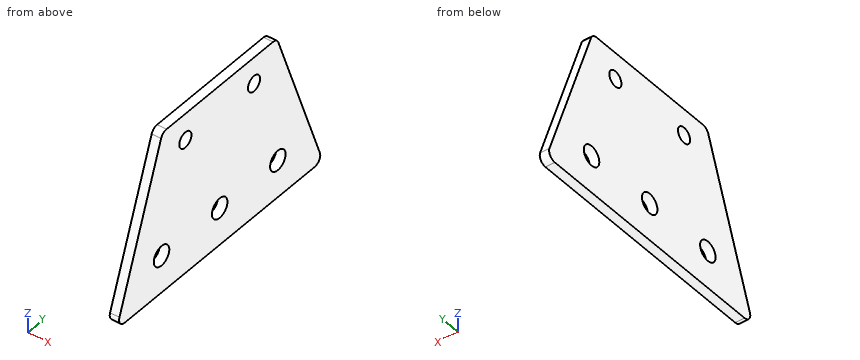
```python
from build123d import *

# Parameters (mm, degrees)
F_1_8_INCH_SHEET_DEPTH     = 1.5875
M5_CLEARANCE_HOLE1_D       = 5.3
F_1_4_IN_CLEARANCE_HOLE1_D = 6.7564
FILLET1_R                  = 2.5


with BuildPart() as part:
    # Sketch1 → 1/8 Inch Sheet (new, symmetric)
    with BuildSketch(Plane(origin=(0, 0, 0), x_dir=(0, 0, -1), z_dir=(1, 0, 0))):
        Polygon((-27.5, 25), (-27.5, -25), (27.5, -45), (27.5, 45), align=None)
    extrude(amount=F_1_8_INCH_SHEET_DEPTH, both=True)

    # M5 Clearance Hole1 (through all)
    with Locations(Plane(origin=(1.5875, 0, 0), x_dir=(0, 0, -1), z_dir=(1, 0, 0))):
        with Locations((-18.5, 15), (-18.5, -15)):
            Hole(M5_CLEARANCE_HOLE1_D / 2)

    # 1/4 in Clearance Hole1 (through all)
    with Locations(Plane(origin=(1.5875, 0, 0), x_dir=(0, 0, -1), z_dir=(1, 0, 0))):
        with Locations((14.8, 25.4), (14.8, 0), (14.8, -25.4)):
            Hole(F_1_4_IN_CLEARANCE_HOLE1_D / 2)

    # Fillet1
    fillet1_edges = [part.edges().sort_by_distance(p)[0] for p in [
        (0, 45, -27.5),
        (0, -45, -27.5),
        (0, -25, 27.5),
        (0, 25, 27.5),
    ]]
    fillet(fillet1_edges, radius=FILLET1_R)


solid = part.part
```
The listing builds one solid part. Answer for the finished solid, in the listing's coordinates (mm). Give positions to 0.01 mm unless a question says otherwise; leave off trailing zeros. Order: outer loops, then holes, each group sorted by start corner. A loop starts at its lowest first (then second) coordinate and runs counter-clockwise, first axis right, second up. Notation, with made-up numbers: (62, -2) -> (89, -2) arc R10 cw to (89, 6) -> close; hole circle Ø5 at (-25, 23.25). An arc over 180 degrees is marked (long way). Write each question's results on one line, items separated by ' | '.
Q1. The part is cut by section A-A, the plane y = -15. Give the vertices of the cut face in (x, z).
Checked values:
outline: (-1.59, -27.5) -> (1.59, -27.5) -> (1.59, 15.85) -> (-1.59, 15.85) -> close; (-1.59, 21.15) -> (1.59, 21.15) -> (1.59, 27.5) -> (-1.59, 27.5) -> close
Q2. Straight lines are drawn through the part: probe 1 along Y at (x, z) = (0, 20.5); probe 2 along Y at (x, z) = (0.45, -14.8); probe 3 along Y at (x, z) = (0.6, 18.5). For each, find the intervals that lie inside material, in ascending order. Write a range as from..to.
Checked values:
probe 1: y = -27.55..-16.74, -13.26..13.26, 16.74..27.55 | probe 2: y = -40.38..-28.78, -22.02..-3.38, 3.38..22.02, 28.78..40.38 | probe 3: y = -28.27..-17.65, -12.35..12.35, 17.65..28.27
Q3. The part is cut by section C-C, the plane z = -14.8. Give the vertices of the cut face in (x, y), and give its area (3 significant figures).
Checked values:
outline: (-1.59, -40.38) -> (1.59, -40.38) -> (1.59, -28.78) -> (-1.59, -28.78) -> close; (-1.59, -22.02) -> (1.59, -22.02) -> (1.59, -3.38) -> (-1.59, -3.38) -> close; (-1.59, 3.38) -> (1.59, 3.38) -> (1.59, 22.02) -> (-1.59, 22.02) -> close; (-1.59, 28.78) -> (1.59, 28.78) -> (1.59, 40.38) -> (-1.59, 40.38) -> close | area: 192 mm^2
Q4. Each of these flat-tipped pins is pushed along its axis until it touches: P1, Ø1.5, axis at x = 0, z = -2, coming from the -Y side; P2, Ø11, axis at y = 0, z = -14.8, coming from the +X side. Where does it stop, or does it pass through?
Checked values:
P1: stops at y = -36 | P2: stops at x = 1.59
Q5. The part is cut by section D-D, the plane y = 0. Give the vertices of the cut face in (x, z).
Checked values:
outline: (-1.59, -27.5) -> (1.59, -27.5) -> (1.59, -18.18) -> (-1.59, -18.18) -> close; (-1.59, -11.42) -> (1.59, -11.42) -> (1.59, 27.5) -> (-1.59, 27.5) -> close
Q6. The part is cut by section B-B, the plane x = 0. Give the vertices of the cut face in (y, z).
Checked values:
outline: (-43.78, -24.15) arc R2.5 ccw to (-41.43, -27.5) -> (41.43, -27.5) arc R2.5 ccw to (43.78, -24.15) -> (25.6, 25.85) arc R2.5 ccw to (23.25, 27.5) -> (-23.25, 27.5) arc R2.5 ccw to (-25.6, 25.85) -> close; hole circle Ø6.76 at (-25.4, -14.8); hole circle Ø5.3 at (-15, 18.5); hole circle Ø6.76 at (0, -14.8); hole circle Ø5.3 at (15, 18.5); hole circle Ø6.76 at (25.4, -14.8)
